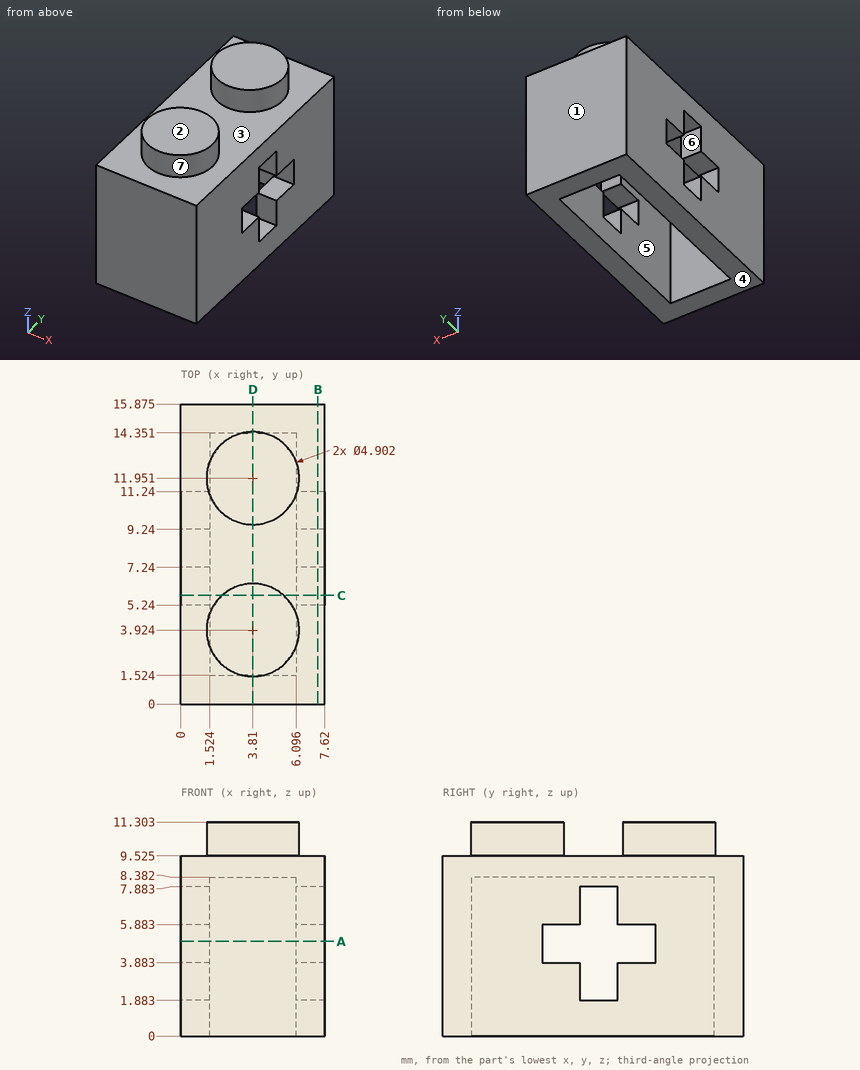
Source: three-view drawing plus pictorial views. Frame: mm from the lowest corner of the part. A direction names the side the tool comes from. Coordinates: 2 decimals unless noted, no trailing zeros. Loops run counter-clockwise (first coordinate to the right, second up) from the corner with the lowest first, then second, coordinate; pieces in that order, holes last. Notation, with made-up numbers: (19.25, -27.5) -> (73.25, -27.5) arc R34 ccw to (73.25, 7.5) -> close; hole circle Ø10 at (-30.75, -16.75). An arc over 180 degrees is marked (long way). Answer in a Markdown table with one row per item. Add a question column.
Q1. Section B-B on x = 7.25. Return the cut outline in (y, z) (1 decimal), and give its area (3 significant figures).
Q2. Contact query for flat-ended pins moving along their axis: pin 1 Ø0.5 at (x, y) = (6.5, 8.5) entering from +Z (3 decimals); pin 2 Ø1 at (x, y) = (3.5, 10.5) entering from -Z. Output: stop coordinate, or through.
Q3. Reachability of the marked faces 4, 5, 6 and 7 from +Z, -Z, +X, -X, +Y, -Y: full face, straight path, thin tool, end or side. Return the list, or none.
Q4. Ray query, line 1 along Y through (x, z) = (5.25, 6) (1 decimal); line 2 along X through (y, z) = (10, 3.5); line 3 along Z through (x, y) = (1, 11) (1 decimal). Return the intervals inside material, ascending.
Q5. Section D-D on x = 3.81. Return the cut outline in (y, z) (1 decimal).
Q6. Section C-C on y = 5.75. Return the cut outline in (x, z) (1 decimal).
Q7. Section A-A on z = 5. Return the cut outline in (x, y) (1 decimal).
Q8. Pull-direction query (Y, two-part tool) for the marked faces 1, 2 and 3; classes: pulls with the +Y half, pulls with the -Y half, needs draft (parallel to the pull), parting line crosses it, or undercut.
Computed values:
| question | item | result |
|---|---|---|
| 1 | outline | (0, 0) -> (15.9, 0) -> (15.9, 9.5) -> (0, 9.5) -> close; hole (5.2, 3.9) -> (7.2, 3.9) -> (7.2, 1.9) -> (9.2, 1.9) -> (9.2, 3.9) -> (11.2, 3.9) -> (11.2, 5.9) -> (9.2, 5.9) -> (9.2, 7.9) -> (7.2, 7.9) -> (7.2, 5.9) -> (5.2, 5.9) -> close |
| 1 | area | 131 mm^2 |
| 2 | pin 1 | stops at z = 9.525 |
| 2 | pin 2 | stops at z = 8.38 |
| 3 | face 4 | -Z, +X, -X, +Y, -Y |
| 3 | face 5 | -Z |
| 3 | face 6 | +X, -X |
| 3 | face 7 | +Z |
| 4 | line 1 | y = 0 to 1.5, 14.4 to 15.9 |
| 4 | line 2 | x = 0 to 1.52, 6.1 to 7.62 |
| 4 | line 3 | z = 0 to 3.9, 5.9 to 9.5 |
| 5 | outline | (0, 0) -> (1.5, 0) -> (1.5, 8.4) -> (14.4, 8.4) -> (14.4, 0) -> (15.9, 0) -> (15.9, 9.5) -> (14.4, 9.5) -> (14.4, 11.3) -> (9.5, 11.3) -> (9.5, 9.5) -> (6.4, 9.5) -> (6.4, 11.3) -> (1.5, 11.3) -> (1.5, 9.5) -> (0, 9.5) -> close |
| 6 | outline | (0, 0) -> (1.5, 0) -> (1.5, 3.9) -> (0, 3.9) -> close; (0, 5.9) -> (1.5, 5.9) -> (1.5, 8.4) -> (6.1, 8.4) -> (6.1, 5.9) -> (7.6, 5.9) -> (7.6, 9.5) -> (5.4, 9.5) -> (5.4, 11.3) -> (2.2, 11.3) -> (2.2, 9.5) -> (0, 9.5) -> close; (6.1, 0) -> (7.6, 0) -> (7.6, 3.9) -> (6.1, 3.9) -> close |
| 7 | outline | (0, 0) -> (7.6, 0) -> (7.6, 5.2) -> (6.1, 5.2) -> (6.1, 1.5) -> (1.5, 1.5) -> (1.5, 5.2) -> (0, 5.2) -> close; (0, 11.2) -> (1.5, 11.2) -> (1.5, 14.4) -> (6.1, 14.4) -> (6.1, 11.2) -> (7.6, 11.2) -> (7.6, 15.9) -> (0, 15.9) -> close |
| 8 | face 1 | pulls with the +Y half |
| 8 | face 2 | needs draft |
| 8 | face 3 | undercut |
